from build123d import *

# Parameters (mm, degrees)
SKETCH_2_R           = 1.6
SKETCH_2_R_2         = 17
SKETCH_2_R_3         = 1.65
EXTRUDE_2_DEPTH      = 1.5
EXTRUDE_3_DEPTH      = 18
EXTRUDE_4_DEPTH      = 10
CUT_EXTRUDE_5_DEPTH  = 116.63018637
SKETCH_10_R          = 3
SKETCH_10_R_2        = 1.65
SKETCH_10_W          = 9
SKETCH_10_H          = 7
CUT_EXTRUDE_4_DEPTH  = 5
EXTRUDE_5_DEPTH      = 18
SKETCH_14_R          = 1.65
CUT_EXTRUDE_6_DEPTH  = 10
CUT_EXTRUDE_7_DEPTH  = 116.63018637
SKETCH_18_W          = 9
SKETCH_18_H          = 5.7
SKETCH_18_W_2        = 24
CUT_EXTRUDE_8_DEPTH  = 10
CUT_EXTRUDE_9_DEPTH  = 10
SKETCH_21_W          = 17.5
SKETCH_21_H          = 7.5
CUT_EXTRUDE_10_DEPTH = 1.2


with BuildPart() as part:
    # 草图2 → 凸台-拉伸2 (new body)
    with BuildSketch(Plane(origin=(0, 0, 0), x_dir=(1, 0, 0), z_dir=(0, 1, 0))):
        Polygon((-42.5, 33.8), (-42.5, 62.8), (-27.5, 62.8), (-27.5, 53.8), (10, 53.8), (10, 62.8), (40, 62.8), (40, 53.8), (77.5, 53.8), (77.5, 62.8), (92.5, 62.8), (92.5, 33.8), (50, 33.8), (50, 0), (0, 0), (0, 33.8), align=None)
        with Locations(Location((-35, 55.312210178, 0), (0, 0, 270))):
            Circle(SKETCH_2_R, mode=Mode.SUBTRACT)
        with Locations(Location((85, 55.312210178, 0), (0, 0, 270))):
            Circle(SKETCH_2_R, mode=Mode.SUBTRACT)
        with Locations(Location((18, 55.312210178, 0), (0, 0, 270))):
            Circle(SKETCH_2_R, mode=Mode.SUBTRACT)
        with Locations(Location((32, 55.312210178, 0), (0, 0, 270))):
            Circle(SKETCH_2_R, mode=Mode.SUBTRACT)
        with Locations(Location((25, 28.8, 0), (0, 0, 270))):
            Circle(SKETCH_2_R_2, mode=Mode.SUBTRACT)
        with Locations(Location((40.5, 44.3, 0), (0, 0, 270))):
            Circle(SKETCH_2_R_3, mode=Mode.SUBTRACT)
        with Locations(Location((40.5, 13.3, 0), (0, 0, 270))):
            Circle(SKETCH_2_R_3, mode=Mode.SUBTRACT)
        with Locations(Location((9.5, 13.3, 0), (0, 0, 270))):
            Circle(SKETCH_2_R_3, mode=Mode.SUBTRACT)
        with Locations(Location((9.5, 44.3, 0), (0, 0, 270))):
            Circle(SKETCH_2_R_3, mode=Mode.SUBTRACT)
    extrude(amount=EXTRUDE_2_DEPTH)

    # 草图6 → 凸台-拉伸3 (add)
    with BuildSketch(Plane(origin=(0, 1.5, 0), x_dir=(1, 0, 0), z_dir=(0, 1, 0))):
        Polygon((10, 53.8), (-27.5, 53.8), (-27.5, 62.8), (-42.5, 62.8), (-42.5, 33.8), (0, 33.8), (0, 0), (50, 0), (50, 33.8), (92.5, 33.8), (92.5, 62.8), (77.5, 62.8), (77.5, 53.8), (40, 53.8), (40, 62.8), (10, 62.8), align=None)
        Polygon((11.2, 52.6), (-28.7, 52.6), (-28.7, 59.8), (-41.3, 59.8), (-41.3, 35), (1.2, 35), (1.2, 2.5), (48.8, 2.5), (48.8, 35), (91.3, 35), (91.3, 60.3), (78.7, 60.3), (78.7, 52.6), (38.8, 52.6), (38.8, 61.6), (11.2, 61.6), align=None, mode=Mode.SUBTRACT)
    extrude(amount=EXTRUDE_3_DEPTH)

    # 草图11 → 凸台-拉伸4 (add)
    with BuildSketch(Plane(origin=(0, 19.5, 0), x_dir=(1, 0, 0), z_dir=(0, 1, 0))):
        Polygon((1.2, 35), (1.2, 2.5), (48.8, 2.5), (48.8, 35), (50, 35), (50, 0), (0, 0), (0, 35), align=None)
    extrude(amount=EXTRUDE_4_DEPTH)

    # 草图12 → 切除-拉伸5 (cut, through all)
    with BuildSketch(Plane.ZY):
        Polygon((-35, 19.5), (-4, 29.5), (-35, 29.5), align=None)
    extrude(amount=-CUT_EXTRUDE_5_DEPTH, mode=Mode.SUBTRACT)

    # 草图10 → 切除-拉伸4 (cut)
    with BuildSketch(Plane.XY):
        with Locations((25, 15.656854249)):
            Circle(SKETCH_10_R)
        with Locations((30.656854249, 21.313708499)):
            Circle(SKETCH_10_R_2)
        with Locations((30.656854249, 10)):
            Circle(SKETCH_10_R_2)
        with Locations((19.343145751, 10)):
            Circle(SKETCH_10_R_2)
        with Locations((19.343145751, 21.313708499)):
            Circle(SKETCH_10_R_2)
        with Locations((8, 22.5)):
            Rectangle(SKETCH_10_W, SKETCH_10_H)
        with Locations((42, 22.5)):
            Rectangle(SKETCH_10_W, SKETCH_10_H)
    extrude(amount=-CUT_EXTRUDE_4_DEPTH, mode=Mode.SUBTRACT)

    # 草图13 → 凸台-拉伸5 (add)
    with BuildSketch(Plane(origin=(0, 1.5, 0), x_dir=(1, 0, 0), z_dir=(0, 1, 0))):
        Polygon((0.316065276, 52.6), (-0.838635262, 52.6), (-11, 35), (-9.845299462, 35), align=None)
        Polygon((-15.154700538, 35), (-14, 35), (-24.161364738, 52.6), (-25.316065276, 52.6), align=None)
        Polygon((59.845299462, 35), (61, 35), (50.838635262, 52.6), (49.683934724, 52.6), align=None)
        Polygon((75.316065276, 52.6), (74.161364738, 52.6), (64, 35), (65.154700538, 35), align=None)
    extrude(amount=EXTRUDE_5_DEPTH)

    # 草图14 → 切除-拉伸6 (cut)
    with BuildSketch(Plane(origin=(0, 0, -62.8), x_dir=(-1, 0, 0), z_dir=(0, 0, -1))):
        with Locations((35, 14.7)):
            Circle(SKETCH_14_R)
        with Locations(Location((-85, 14.7, 0), (0, 0, 180))):
            Circle(SKETCH_14_R)
        with Locations((-25, 14.7)):
            Circle(SKETCH_14_R)
    extrude(amount=-CUT_EXTRUDE_6_DEPTH, mode=Mode.SUBTRACT)

    # 草图17 → 切除-拉伸7 (cut, through all)
    with BuildSketch(Plane.ZY):
        Polygon((-7, 21.177065656), (-27, 14.725452753), (-27, 7.725452753), (-7, 7.725452753), align=None)
    extrude(amount=-CUT_EXTRUDE_7_DEPTH, mode=Mode.SUBTRACT)

    # 草图18 → 切除-拉伸8 (cut)
    with BuildSketch(Plane(origin=(0, 0, -62.8), x_dir=(-1, 0, 0), z_dir=(0, 0, -1))):
        with Locations((-85, 6.85)):
            Rectangle(SKETCH_18_W, SKETCH_18_H)
        with Locations((-25, 6.85)):
            Rectangle(SKETCH_18_W_2, SKETCH_18_H)
        with Locations((35, 6.85)):
            Rectangle(SKETCH_18_W, SKETCH_18_H)
    extrude(amount=-CUT_EXTRUDE_8_DEPTH, mode=Mode.SUBTRACT)

    # 草图20 → 切除-拉伸9 (cut)
    with BuildSketch(Plane(origin=(0, 1.5, 0), x_dir=(1, 0, 0), z_dir=(0, 1, 0))):
        Polygon((-12.5, 40.401923789), (-7.766838493, 48.6), (-17.233161507, 48.6), align=None)
        Polygon((62.5, 40.401923789), (67.233161507, 48.6), (57.766838493, 48.6), align=None)
        Polygon((-36.3, 50.373953839), (-33.7, 50.373953839), (-33.7, 47.6), (-28.202816622, 47.6), (-23.814954576, 40), (-36.3, 40), align=None)
        Polygon((86.3, 40), (73.814954576, 40), (78.202816622, 47.6), (83.7, 47.6), (83.7, 50.373953839), (86.3, 50.373953839), align=None)
    extrude(amount=-CUT_EXTRUDE_9_DEPTH, mode=Mode.SUBTRACT)

    # 草图21 → 切除-拉伸10 (cut)
    with BuildSketch(Plane(origin=(0, 0, -53.8), x_dir=(-1, 0, 0), z_dir=(0, 0, -1))):
        with Locations((11.75, 9.75)):
            Rectangle(SKETCH_21_W, SKETCH_21_H)
        with Locations((-61.75, 9.75)):
            Rectangle(SKETCH_21_W, SKETCH_21_H)
    extrude(amount=-CUT_EXTRUDE_10_DEPTH, mode=Mode.SUBTRACT)


solid = part.part
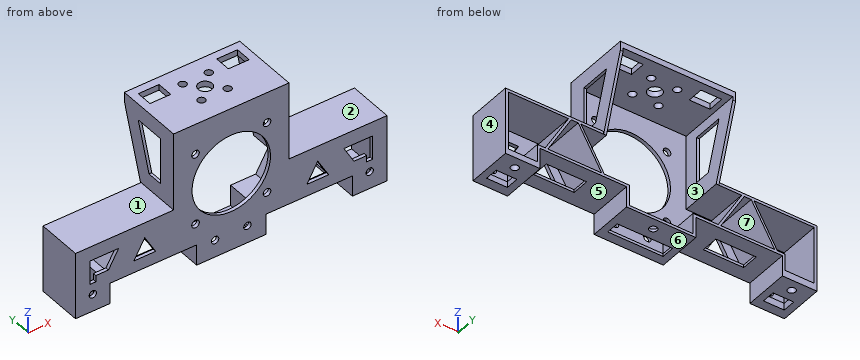
Design review of the part built by this model. Coordinates are the model's own, in mm. Face numbers are marked on the shaded views. A direction names the side the tool comes from. Coordinates: 2 decimals unless noted, no trailing zeros. Loops run counter-clockwise (first coordinate to the right, second up) from the corner with the lowest first, then second, coordinate; pieces in that order, holes last. Notation, with made-up numbers: M 41.25,73 L 56.25,73 A12 ccw 56.25,80 Z; hole C 74,-35 d1. An arc over 180 degrees is marked long. Answer as CSV lines item,"result".
Item 1: Add section C-C on x = 85. State the section outline as (y, z) points, plus the area to 3 significant figures.
Answer list:
outline,"M 0,-62.8 L 4,-62.8 L 4,-60.3 L 1.5,-60.3 L 1.5,-56.91 L 0,-56.91 Z; M 0,-53.71 L 1.5,-53.71 L 1.5,-50.37 L 0,-50.37 Z; M 0,-40 L 1.5,-40 L 1.5,-35 L 19.5,-35 L 19.5,-33.8 L 0,-33.8 Z; M 9.7,-62.8 L 13.05,-62.8 L 13.05,-60.3 L 9.7,-60.3 Z; M 16.35,-62.8 L 19.5,-62.8 L 19.5,-60.3 L 16.35,-60.3 Z"
area,"67.2 mm²"
Item 2: For probe 1 along Y at (x, z) = (25, -62.05); probe 2 along Y at (x, z) = (25, -1); probe 3 along Z at (x, y) = (-27, 13.75), list the stretches that pass through material, from the lowest coordinate up.
Answer list:
probe 1,"0 to 4, 9.7 to 13.05, 16.35 to 19.5"
probe 2,"0 to 12.66, 18.66 to 29.5"
probe 3,"-53.8 to -52.6, -35 to -33.8"
Item 3: Add section A-A on x = -35. State the section outline as (y, z) points, plus the area to 3 significant figures.
Answer list:
outline,"M 0,-62.8 L 4,-62.8 L 4,-59.8 L 1.5,-59.8 L 1.5,-56.91 L 0,-56.91 Z; M 0,-53.71 L 1.5,-53.71 L 1.5,-50.37 L 0,-50.37 Z; M 0,-40 L 1.5,-40 L 1.5,-35 L 19.5,-35 L 19.5,-33.8 L 0,-33.8 Z; M 9.7,-62.8 L 13.05,-62.8 L 13.05,-59.8 L 9.7,-59.8 Z; M 16.35,-62.8 L 19.5,-62.8 L 19.5,-59.8 L 16.35,-59.8 Z"
area,"71.7 mm²"
Item 4: The part is to be moulded in two halves that separate along X. For the marked faces 4, 5, 6 and 7, say which applies: pulls with the +X half, pulls with the -X half, needs draft (parallel to the pull), parting line crosses it, or undercut.
Answer list:
face 4,"pulls with the +X half"
face 5,"undercut"
face 6,"needs draft"
face 7,"undercut"
Item 5: Add section D-D on z = -44. Count the separate pieces of the cut face and the enclosed holes in it, plus the area to 3 significant figures.
Answer list:
separate pieces,"8"
enclosed holes,"0"
area,"253 mm²"
Item 6: Machinability: for the marked faces 1, 2 and 3, which of the approach directions +Z, -Z, +X, -X, +Y, -Y give a long, thin tool a straight path to every point of the face, cutting with its end or side? Answer none if there is none.
Answer list:
face 1,"+Z, -X, +Y, -Y"
face 2,"+Z, +X, +Y, -Y"
face 3,"+Y"
Item 7: For P1, Ø23, axis at x = 17.5, z = -47, coming from the +Y side; P2, Ø1.6, axis at x = 84.5, y = 0.5, coming from the +Z side; P3, Ø5, axis at y = 14, z = -28.5, coming from the +X side; P4, Ø10, axis at x = 21.5, z = -19, coming from the -Y side, all flat-tipped, find the tip position at first contact; note any pin that passes through.
Answer list:
P1,"y = 19.5"
P2,"z = -33.8"
P3,"x = 50"
P4,"through"
Item 8: Add section B-B on z = -31.5. State the section outline as (x, y) points, plus the area to 3 significant figures.
Answer list:
outline,"M 0,0 L 8.22,0 L 8.22,1.5 L 1.2,1.5 L 1.2,20.63 L 0,20.63 Z; M 41.78,0 L 50,0 L 50,20.63 L 48.8,20.63 L 48.8,1.5 L 41.78,1.5 Z"
area,"70.6 mm²"
